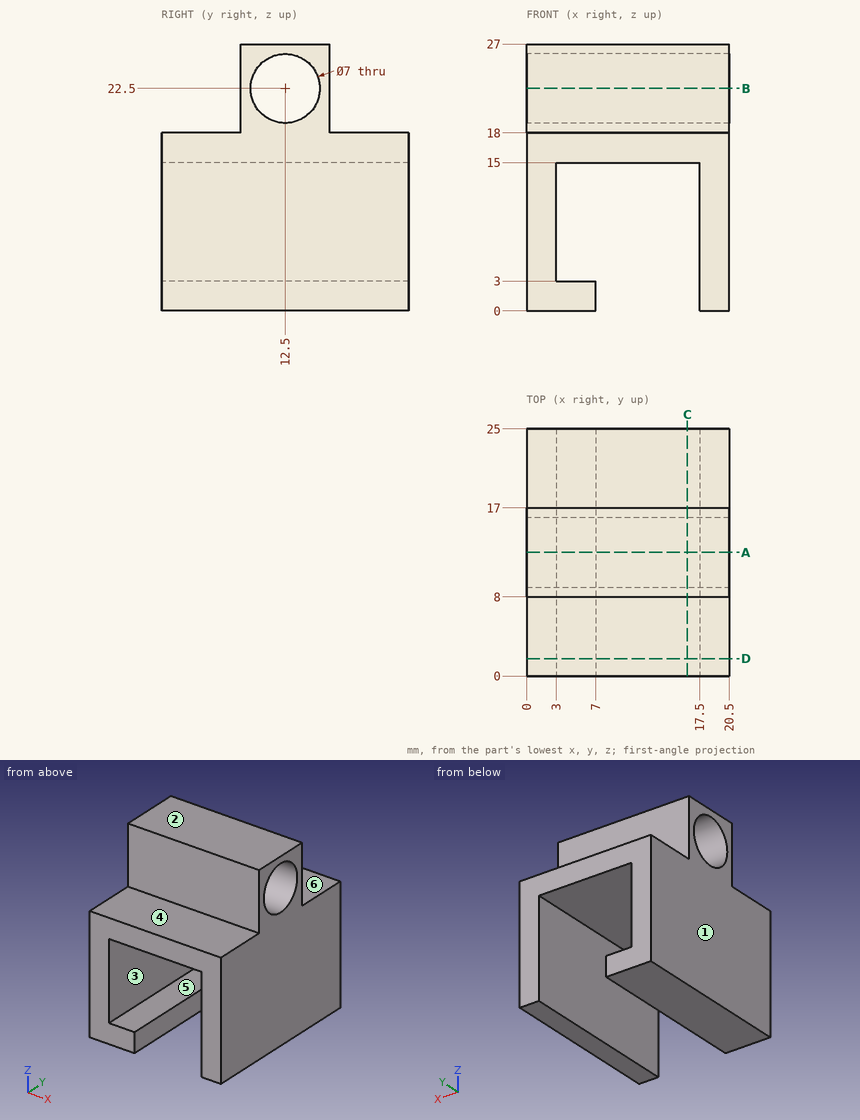
Can you work these out from the drawing? Everything is in mm from the part's minimum corner. A direction names the side the tool comes from. Round coordinates to 2 decimals unless told otherwise and drop trailing zeros. Order: outer loops, then holes, each group sorted by start corner. A loop starts at its lowest first (then second) coordinate and runs counter-clockwise, first axis right, second up.
(1) If we section it at D-D (y = 1.75): Please give me the cut outline in (x, z), plus the area to 4 significant figures.
Results are:
outline: (0, 0) - (7, 0) - (7, 3) - (3, 3) - (3, 15) - (17.5, 15) - (17.5, 0) - (20.5, 0) - (20.5, 18) - (0, 18) - close
area: 163.5 mm2
(2) If we section it at A-A (y = 12.5): Please give me the cut outline in (x, z).
Results are:
outline: (0, 0) - (7, 0) - (7, 3) - (3, 3) - (3, 15) - (17.5, 15) - (17.5, 0) - (20.5, 0) - (20.5, 19) - (0, 19) - close; (0, 26) - (20.5, 26) - (20.5, 27) - (0, 27) - close
(3) If we section it at C-C (x = 16.25): Please give me the cut outline in (y, z), plus the area to 3 significant figures.
Results are:
outline: (0, 15) - (25, 15) - (25, 18) - (17, 18) - (17, 27) - (8, 27) - (8, 18) - (0, 18) - close; hole circle Ø7 at (12.5, 22.5)
area: 118 mm2
(4) On a 3-axis mill with a long thin cutter (end or side, diameter ignored), from which of +Z, -Z, +X, -X, +Y, -Y can I reach the whole of each face in a straight line? I mean the marked faces 4, 5 and 6. Say none if no direction works.
Results are:
face 4: +Z, +X, -X, -Y
face 5: +Y, -Y
face 6: +Z, +X, -X, +Y
(5) I'm going to push flat-ended pins straight in: pin 1 (10 mm diameter, centred on x = 11.5, z = 24, fed in from -Y); pin 2 (2.5 mm diameter, centred on x = 14.5, y = 5, fed in from +Z). Where does each tip first touch, or does it pass through?
Results are:
pin 1: stops at y = 8
pin 2: stops at z = 18
(6) If I drill on L1, parallel to Z at x = 5.5, y = 12.5; L2, parallel to X at y = 8.5, z = 6; L3, parallel to Z at x = 14, y = 12.5, over which ranges is the centre line in solid material (lowest first)?
Results are:
L1: z = 0 to 3, 15 to 19, 26 to 27
L2: x = 0 to 3, 17.5 to 20.5
L3: z = 15 to 19, 26 to 27
(7) If we section it at B-B (z = 22.5): Please give me the cut outline in (x, y).
Results are:
outline: (0, 8) - (20.5, 8) - (20.5, 9) - (0, 9) - close; (0, 16) - (20.5, 16) - (20.5, 17) - (0, 17) - close
(8) We'd pull the mould along X, two halves only. Please class the marked faces 1, 2 and 3: +X half, -X half, draft (parallel to the pull), parting line (faces both ways), or undercut.
Results are:
face 1: -X half
face 2: draft
face 3: undercut
